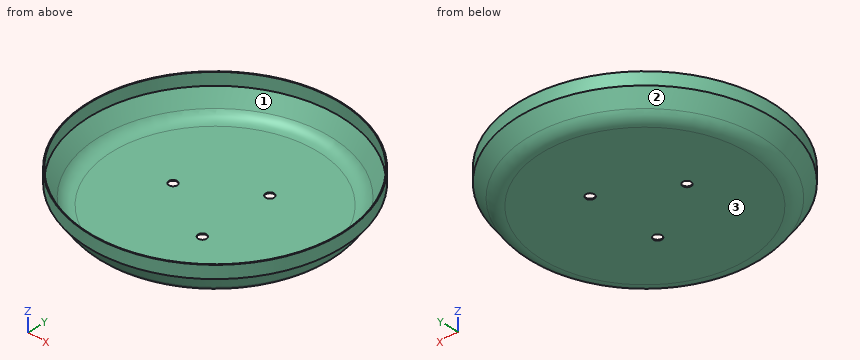
Autodesk Inventor part; units mm, degrees
ref_plane "YZ Plane" through (0, 0, 0) normal (1, 0, 0) x (0, 1, 0)
ref_plane "XZ Plane" through (0, 0, 0) normal (0, 1, 0) x (-1, 0, 0)
ref_plane "XY Plane" through (0, 0, 0) normal (0, 0, 1) x (1, 0, 0)
sketch "Sketch2" plane through (0, 0, 0) normal (0, 1, 0) x (-1, 0, 0)
  line L0 (0, 0) -> (-610.4174, 0)
  line L1 (-692.3326, 42.6424) -> (-750, 125)
  line L2 (-750, 200) -> (0, 200)
  line L3 (0, 200) -> (0, 0)
  arc A0 (-692.3326, 42.6424) -> (-610.4174, 0) centre (-610.4174, 100) ccw
  line L4 (-750, 200) -> (-750, 125)
  dimension "d0" = 100
  dimension "d1" = 200
  dimension "d2" = 750
  dimension "d3" = 125
  dimension "d4" = 75
revolve "Revolution1" add sketch "Sketch2" angle 360 about axis through (0, 0, 200) along (0, 0, -1)
shell "Shell1" thickness 5 removed faces 1 at (-44.9023, -186.6904, 200)
sketch "Sketch4" plane through (0, 0, 0) normal (0, 0, -1) x (-1, 0, 0)
  line L0 (1050, 0) -> (-1050, 0) construction
  line L1 (0, -1050) -> (0, 1050) construction
  circle A0 centre (-125, -216.5064) radius 25
  line L2 (-125, -216.5064) -> (0, 0) construction
  circle A1 centre (250, 0) radius 25
  circle A2 centre (-125, 216.5064) radius 25
  dimension "d8" = 50
  dimension "d9" = 60
  dimension "d10" = 250
  dimension "d13" = 360
extrude "Extrusion1" cut sketch "Sketch4" against normal through all
properties part number "Saucer"
Source: CAD feature listing. Evaluate the final solid. Frame: model axes, mm. Face numbers are marked on the shaded views. Coordinates: 2 decimals unless noted, no trailing zeros. Order: outer loops, then holes, each group sorted by start corner. A loop starts at its lowest first (then second) coordinate and runs counter-clockwise, first axis right, second up.
Item 1: First-contact query: P1, Ø1.5, axis at y = -131, z = 126, coming from the -X side; P2, Ø12, axis at x = 231, z = 45, coming from the -Y side; P3, Ø10, axis at y = -87, z = 50, coming from the -X side. Flat tips, straight axial feed; report the tip coordinate or a pass-through.
Output values:
P1: stops at x = -738.6
P2: stops at y = -659.33
P3: stops at x = -695.62
Item 2: Cut plane A-A (y = 0). Return loops of the section in (x, z), plus the area to 3 significant figures.
Output values:
outline: (-750, 125) - (-692.33, 42.64) arc R100 ccw to (-610.42, 0) - (-275, 0) - (-275, 5) - (-610.42, 5) arc R95 cw to (-688.24, 45.51) - (-745, 126.58) - (-745, 200) - (-750, 200) - close; (-225, 0) - (610.42, 0) arc R100 ccw to (692.33, 42.64) - (750, 125) - (750, 200) - (745, 200) - (745, 126.58) - (688.24, 45.51) arc R95 cw to (610.42, 5) - (-225, 5) - close
area: 8,530 mm2
Item 3: Material intervals for line 1 (Y direction, x = 0, z = 183.5); line 2 (Z direction, x = 348, y = 427); line 3 (X direction, y = -349, z = 135), sorted ascending.
Output values:
line 1: y = -750 to -745, 745 to 750
line 2: z = 0 to 5
line 3: x = -663.85 to -658.2, 658.2 to 663.85
Item 4: Cut plane B-B (x = 0). Return loops of the section in (y, z), plus the area to 3 significant figures.
Output values:
outline: (-750, 125) - (-692.33, 42.64) arc R100 ccw to (-610.42, 0) - (610.42, 0) arc R100 ccw to (692.33, 42.64) - (750, 125) - (750, 200) - (745, 200) - (745, 126.58) - (688.24, 45.51) arc R95 cw to (610.42, 5) - (-610.42, 5) arc R95 cw to (-688.24, 45.51) - (-745, 126.58) - (-745, 200) - (-750, 200) - close
area: 8,780 mm2
Item 5: Pull-direction query (X, two-part tool) for the marked faces 1, 2 and 3; classes: pulls with the +X half, pulls with the -X half, needs draft (parallel to the pull), parting line crosses it, or undercut.
Output values:
face 1: undercut
face 2: parting line crosses it
face 3: needs draft
